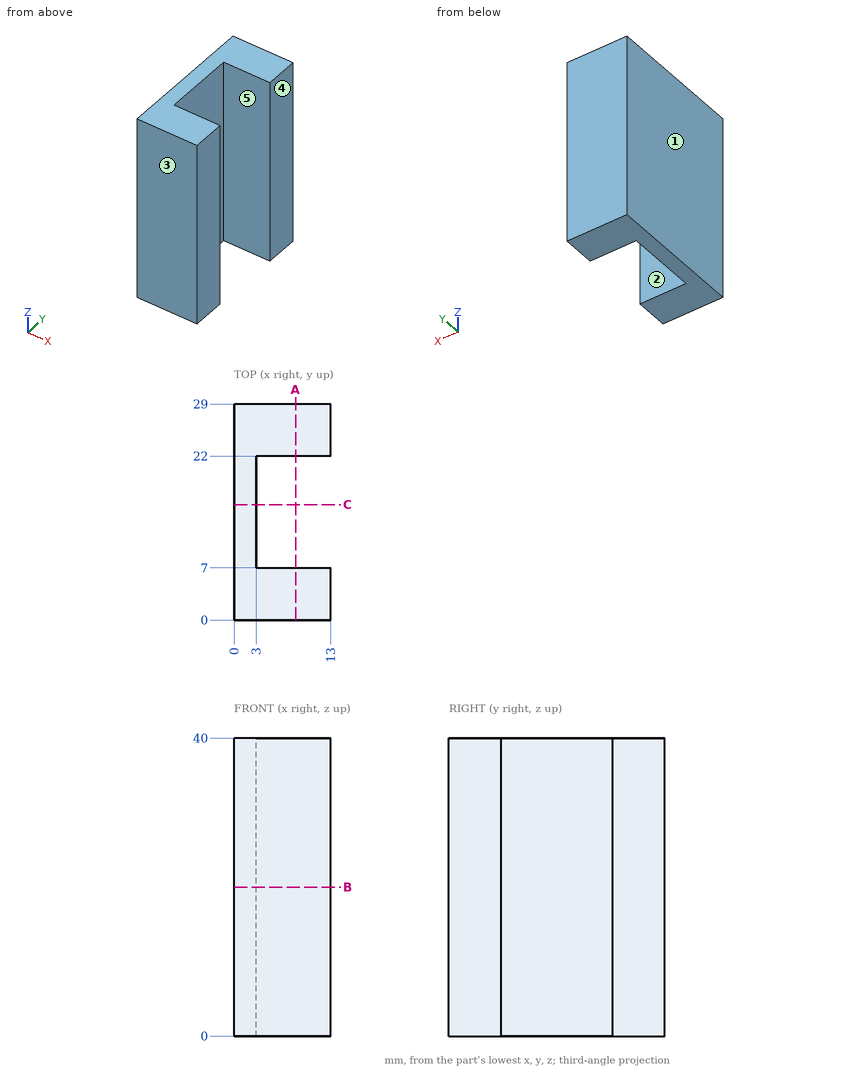
Answer from the drawing. Dimensions are ordinates in mm from the lowest x, y and z of the part. A direction names the side the tool comes from. Give positions to 0.01 mm unless a question says otherwise; leave off trailing zeros. Write each loop counter-clockwise with the first axis right and the second up, starting at its lowest first coordinate (ties: lowest second). Pieces come first, ordered by that corner, then holes. Notation, with made-up numbers: (-13, 41.25) -> (18, 41.25) arc R9 cw to (18, 47.25) -> close; hole circle Ø6 at (68, 61.25). An arc over 180 degrees is marked (long way). Use a Markdown table: item, result.
(1) Section A-A, the plane x = 8.25 is taken. Determine the outline of the cut face in (y, z).
Return value:
| item | result |
|---|---|
| outline | (0, 0) -> (7, 0) -> (7, 40) -> (0, 40) -> close; (22, 0) -> (29, 0) -> (29, 40) -> (22, 40) -> close |
(2) For the marked faces 1 and 2, determine the directions among +Z, -Z, +X, -X, +Y, -Y from which every point of the face is accessible in a straight line to the end or side of a thin tool.
Return value:
| item | result |
|---|---|
| face 1 | +Z, -Z, -X, +Y, -Y |
| face 2 | +Z, -Z, +X |
(3) Find the intervals of material crossed by probe 1 along Y at (x, z) = (12.25, 38.5); probe 2 along X at (y, z) = (11.5, 18), in increasing order. Write a range as from..to.
Return value:
| item | result |
|---|---|
| probe 1 | 0..7, 22..29 |
| probe 2 | 0..3 |
(4) A flat-ended cylindrical pin translates along its axis: P1, Ø12, axis at y = 13.5, z = 20, coming from the +X side. Find the tip coordinate at first contact, or state that the pin passes through.
Return value:
| item | result |
|---|---|
| P1 | x = 3 |
(5) Section C-C, the plane y = 15.5 is taken. Determine the outline of the cut face in (x, z), then the cut area to 3 significant figures.
Return value:
| item | result |
|---|---|
| outline | (0, 0) -> (3, 0) -> (3, 40) -> (0, 40) -> close |
| area | 120 mm2 |
(6) Section B-B, the plane z = 20 is taken. Determine the outline of the cut face in (x, y), then the cut area to 3 significant figures.
Return value:
| item | result |
|---|---|
| outline | (0, 0) -> (13, 0) -> (13, 7) -> (3, 7) -> (3, 22) -> (13, 22) -> (13, 29) -> (0, 29) -> close |
| area | 227 mm2 |
(7) Determine the mould class of the marked faces 3, 4 and 5 for opening direction Y: released by +Y, released by -Y, zero draft, split by the parting line, or undercut.
Return value:
| item | result |
|---|---|
| face 3 | released by -Y |
| face 4 | zero draft |
| face 5 | undercut |
